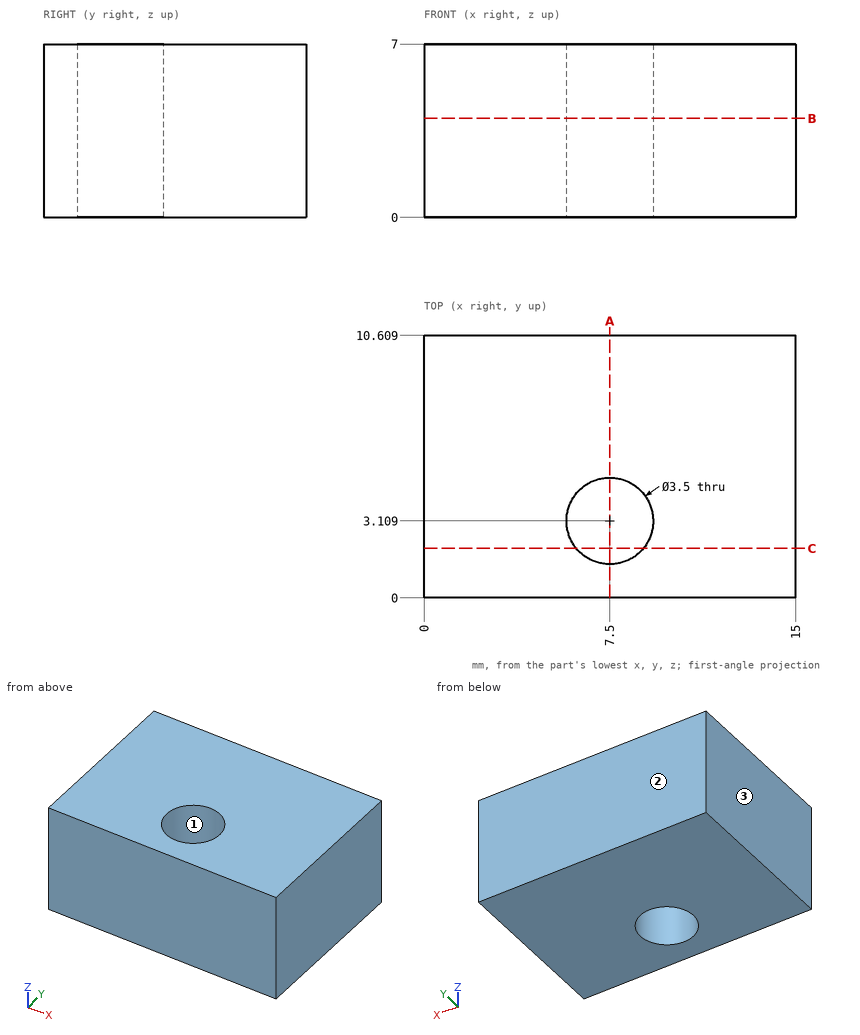
Source: three-view drawing plus pictorial views. Frame: mm from the lowest corner of the part. Coordinates: 2 decimals unless noted, no trailing zeros. Order: outer loops, then holes, each group sorted by start corner. A loop starts at its lowest first (then second) coordinate and runs counter-clockwise, first axis right, second up.
1) Section B-B (z = 4). Return loops of the section in (x, y).
Result sheet:
outline: (0, 0) - (15, 0) - (15, 10.61) - (0, 10.61) - close; hole circle Ø3.5 at (7.5, 3.11)
2) Section A-A (x = 7.5). Return loops of the section in (y, z).
Result sheet:
outline: (0, 0) - (1.36, 0) - (1.36, 7) - (0, 7) - close; (4.86, 0) - (10.61, 0) - (10.61, 7) - (4.86, 7) - close
3) Draft query along Y for the marked faces 1, 2 and 3. Return one class per face: released by +Y, released by -Y, zero draft, split by the parting line, or undercut.
Result sheet:
face 1: undercut
face 2: released by +Y
face 3: zero draft
4) Section C-C (y = 2). Return loops of the section in (x, z).
Result sheet:
outline: (0, 0) - (6.15, 0) - (6.15, 7) - (0, 7) - close; (8.85, 0) - (15, 0) - (15, 7) - (8.85, 7) - close
5) Ray query, probe 1 along X at (y, z) = (3, 6.5); probe 2 along X at (y, z) = (4.25, 0.5); probe 3 along Y at (x, z) = (7.75, 3). Return the intervals inside material, ascending.
Result sheet:
probe 1: x = 0 to 5.75, 9.25 to 15
probe 2: x = 0 to 6.17, 8.83 to 15
probe 3: y = 0 to 1.38, 4.84 to 10.61
